Geometry check sheet. Reference: the model listing, model coordinates, mm. Give positions to 0.01 mm unless a question says otherwise; leave off trailing zeros. Write each loop counter-clockwise with the first axis right and the second up, starting at its lowest first coordinate (ties: lowest second). Pieces come first, ordered by that corner, then holes. Notation, with made-up numbers: (9, 74) - (47, 74) arc R24 cw to (47, 91) - close; hole circle Ø9 at (-20, 23.5). An arc over 180 degrees is marked (long way). One line per question, with ' | ' between items. Start each with the question number.
Q1. Section check D-D on z = 8.25. Record the boundary of the cut face in (x, y), and give its area (3 significant figures).
Q2. Section check C-C on y = 2.3. Record the boundary of the cut face in (x, z), and give its area (3 significant figures).
Q3. Section check A-A on z = 0. Record the boundary of the cut face in (x, y), and give its area (4 significant figures).
Q4. Section check B-B on x = 0. Record the boundary of the cut face in (y, z), and give its area (4 significant figures).
Q5. Gauge pin test, flat end, axial feed: P1, Ø5, axis at x = 10, z = -9.5, coming from the +Y side. Record the tip position at first contact, or that the pin passes through.
Q6. Thickness scan on L1, parallel to X at y = 2.15, z = 0; L2, parallel to Z at x = 0.5, y = 2.6; L3, parallel to Z at x = 0.25, y = 2.85. Record the ranges inside material, lowest first. Write a range as [from, to].
```python
from build123d import *

# Parameters (mm, degrees)
SKETCH1_R           = 10.5
SKETCH1_R_2         = 1
BOSS_EXTRUDE1_DEPTH = 1.5
SKETCH2_R           = 13.15
SKETCH2_R_2         = 10.5
SKETCH2_R_3         = 1
BOSS_EXTRUDE2_DEPTH = 1.5
SKETCH4_R           = 10.5
CUT_EXTRUDE1_DEPTH  = 1.5


with BuildPart() as part:
    # Sketch1 → Boss-Extrude1 (new body)
    with BuildSketch(Plane(origin=(0, 0, 0), x_dir=(1, 0, 0), z_dir=(0, 1, 0))):
        with Locations(Location((0, 0, 0), (0, 0, 270))):
            Circle(SKETCH1_R)
        with Locations(Location((0, 0, 0), (0, 0, 270))):
            Circle(SKETCH1_R_2, mode=Mode.SUBTRACT)
    extrude(amount=BOSS_EXTRUDE1_DEPTH)

    # Sketch2 → Boss-Extrude2 (add)
    with BuildSketch(Plane(origin=(0, 1.5, 0), x_dir=(1, 0, 0), z_dir=(0, 1, 0))):
        with Locations(Location((0, 0, 0), (0, 0, 270))):
            Circle(SKETCH2_R)
        with Locations(Location((0, 0, 0), (0, 0, 270))):
            Circle(SKETCH2_R_2, mode=Mode.SUBTRACT)
        with Locations(Location((0, 0, 0), (0, 0, 270))):
            Circle(SKETCH2_R_2)
        with Locations(Location((0, 0, 0), (0, 0, 270))):
            Circle(SKETCH2_R_3, mode=Mode.SUBTRACT)
    extrude(amount=BOSS_EXTRUDE2_DEPTH)

    # Sketch4 → Cut-Extrude1 (cut)
    with BuildSketch(Plane.XZ):
        Circle(SKETCH4_R)
    extrude(amount=-CUT_EXTRUDE1_DEPTH, mode=Mode.SUBTRACT)


solid = part.part
```
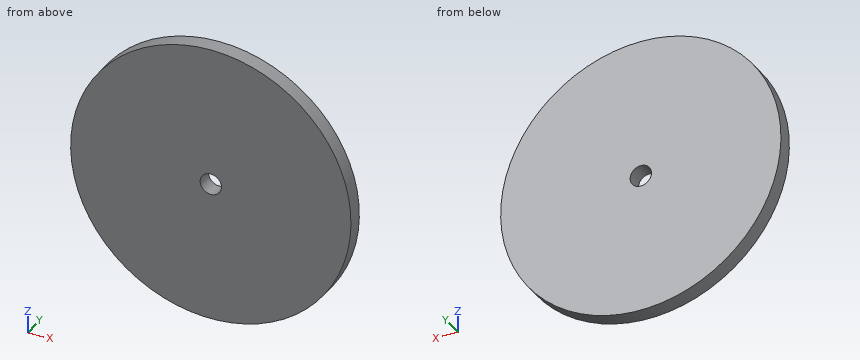
Working result:
1) outline: (-10.24, 1.5) - (10.24, 1.5) - (10.24, 3) - (-10.24, 3) - close | area: 30.7 mm2
2) outline: circle Ø26.3 at (0, 0); hole circle Ø2 at (0, 0) | area: 540 mm2
3) outline: (-13.15, 1.5) - (-1, 1.5) - (-1, 3) - (-13.15, 3) - close; (1, 1.5) - (13.15, 1.5) - (13.15, 3) - (1, 3) - close | area: 36.45 mm2
4) outline: (1.5, -13.15) - (3, -13.15) - (3, -1) - (1.5, -1) - close; (1.5, 1) - (3, 1) - (3, 13.15) - (1.5, 13.15) - close | area: 36.45 mm2
5) P1: stops at y = 3
6) L1: x = [-13.15, -1], [1, 13.15] | L2: z = [-13.14, -0.87], [0.87, 13.14] | L3: z = [-13.15, -0.97], [0.97, 13.15]
